from build123d import *

# Parameters (mm, degrees)
F0_R     = 1.5
F1_DEPTH = 3
F2_R     = 3


# Not quite as in the source:
# - a feature names something its author has since deleted; it is built from what else it names


with BuildPart() as f1:
    # F0 (on Top) → F1 (new body)
    with BuildSketch(Plane.XY):
        with BuildLine():
            ThreePointArc((-14.1339745962, -7.1602540378), (-14.1339745962, -8.1602540378), (-13.2679491924, -8.6602540378))
            Line((-13.2679491924, -8.6602540378), (13.2679491924, -8.6602540378))
            ThreePointArc((13.2679491924, -8.6602540378), (14.1339745962, -8.1602540378), (14.1339745962, -7.1602540378))
            Line((14.1339745962, -7.1602540378), (2.096494358, 13.6892733298))
            ThreePointArc((2.096494358, 13.6892733298), (0.0937033826, 18.2173425378), (-2.2128362603, 13.8361945924))
            Line((-2.2128362603, 13.8361945924), (-14.1339745962, -7.1602540378))
        make_face()
        with BuildLine():
            Line((-4.9019237886, 4.3301270189), (4.9019237886, 4.3301270189))
            ThreePointArc((4.9019237886, 4.3301270189), (6.2009618943, 3.5801270189), (6.2009618943, 2.0801270189))
            Line((6.2009618943, 2.0801270189), (1.2990381057, -6.4102540378))
            ThreePointArc((1.2990381057, -6.4102540378), (0, -7.1602540378), (-1.2990381057, -6.4102540378))
            Line((-1.2990381057, -6.4102540378), (-6.2009618943, 2.0801270189))
            ThreePointArc((-6.2009618943, 2.0801270189), (-6.2009618943, 3.5801270189), (-4.9019237886, 4.3301270189))
        make_face(mode=Mode.SUBTRACT)
        with Locations((0, 15.468939424)):
            Circle(F0_R, mode=Mode.SUBTRACT)
    extrude(amount=F1_DEPTH)

    # F2
    f2_edges = [f1.edges().sort_by_distance(p)[0] for p in [
        (-2.212836, 13.836195, 1.5),
        (2.096494, 13.689273, 1.5),
    ]]
    fillet(f2_edges, radius=F2_R)


solid = f1.part
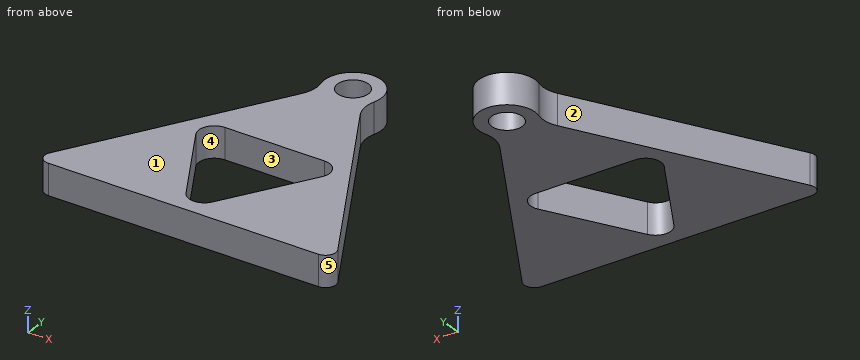
Geometry check sheet. Reference: the model listing, model coordinates, mm. Face numbers are marked on the shaded views. A direction names the side the tool comes from. Give positions to 0.01 mm unless a question says otherwise; leave off trailing zeros. Loops run counter-clockwise (first coordinate to the right, second up) from the corner with the lowest first, then second, coordinate; pieces in that order, holes last.
(1) Release check for a two-part mould opening along X. For the marked faces 1, 2 and 3 record: released by +X, released by -X, zero draft, split by the parting line, or undercut.
From the geometry:
face 1: zero draft
face 2: released by -X
face 3: undercut
(2) Section check B-B on z = 0.8. Record the cut outline in (x, y), then the cut area to 3 significant figures.
From the geometry:
outline: (-14.13, -7.16) arc R1 ccw to (-13.27, -8.66) - (13.27, -8.66) arc R1 ccw to (14.13, -7.16) - (2.9, 12.29) arc R3 cw to (2.63, 14.67) arc R2.75 ccw (long way) to (-2.66, 14.77) arc R3 cw to (-2.95, 12.53) - close; hole (-6.2, 2.08) - (-1.3, -6.41) arc R1.5 ccw to (1.3, -6.41) - (6.2, 2.08) arc R1.5 ccw to (4.9, 4.33) - (-4.9, 4.33) arc R1.5 ccw to start; hole circle Ø3 at (0, 15.47)
area: 304 mm2
(3) Section check A-A on x = 0. Record the cut outline in (y, z), then the cut area to 3 significant figures.
From the geometry:
outline: (-8.66, 0) - (-7.16, 0) - (-7.16, 3) - (-8.66, 3) - close; (4.33, 0) - (13.97, 0) - (13.97, 3) - (4.33, 3) - close; (16.97, 0) - (18.22, 0) - (18.22, 3) - (16.97, 3) - close
area: 37.2 mm2
(4) Section check D-D on y = 9.75. Record the cut outline in (x, z), then the cut area to 3 significant figures.
From the geometry:
outline: (-4.53, 0) - (4.37, 0) - (4.37, 3) - (-4.53, 3) - close
area: 26.7 mm2
(5) Section check C-C on x = -3.5. Record the cut outline in (y, z), then the cut area to 3 significant figures.
From the geometry:
outline: (-8.66, 0) - (-2.6, 0) - (-2.6, 3) - (-8.66, 3) - close; (4.33, 0) - (11.57, 0) - (11.57, 3) - (4.33, 3) - close
area: 39.9 mm2
(6) Depth check by flat-ended pin: pin 1 Ø2 at (x, y) = (6.5, 10) entering from -Z; pin 2 Ø1.5 at (y, z) = (9.5, 2) entering from +X; pin 3 Ø1.5 at (y, z) = (7, 2) entering from -X. Enter the tip coordinate at first touch or a pass-through.
From the geometry:
pin 1: passes through
pin 2: stops at x = 4.95
pin 3: stops at x = -6.52
(7) Thickness scan on L1, parallel to Y at x = 0, z = 2.15; L2, parallel to X at y = -4, z = 0.65; L3, parallel to X at y = -0.75, z = 1.55. Record the ranges inside material, lowest first.
From the geometry:
L1: y = -8.66 to -7.16, 4.33 to 13.97, 16.97 to 18.22
L2: x = -12.34 to -2.69, 2.69 to 12.31
L3: x = -10.49 to -4.57, 4.57 to 10.43
(8) Set-up check for the marked faces 4 and 5: record each of +Z, -Z, +X, -X, +Y, -Y from which the full face is reachable in a straight line by a thin tool's end or side.
From the geometry:
face 4: +Z, -Z
face 5: +Z, -Z, +X
